Work out the finished part from the listing and answer in its coordinate system (mm). A direction names the side the tool comes from. Give positions to 0.01 mm unless a question says otherwise; leave off trailing zeros. Loops run counter-clockwise (first coordinate to the right, second up) from the corner with the lowest first, then second, coordinate; pieces in that order, holes last. Notation, with made-up numbers: (-22, 57.25) - (-2, 57.25) arc R14 ccw to (-2, 67.25) - close; hole circle Ø10 at (61.25, 20.25). An arc over 180 degrees is marked (long way). One line per item, written item: value.
from build123d import *

# Parameters (mm, degrees)
CYLINDER_R      = 1.65
CYLINDER_DEPTH  = 30
PAD005_DEPTH    = 1.05
PAD001_DEPTH    = 3.3
POCKET004_DEPTH = 28.001
PAD002_DEPTH    = 0.5
FILLET_R        = 0.7
FILLET002_R     = 1


with BuildPart() as black_led_base:
    # Cylinder → Cylinder (join)
    with BuildSketch(Plane(origin=(-6, 0, -15), x_dir=(1, 0, 0), z_dir=(0, 0, 1))):
        Circle(CYLINDER_R)
    extrude(amount=CYLINDER_DEPTH)


with BuildPart() as obj1:
    # Sketch016 → Pad005 (new body, symmetric)
    with BuildSketch(Plane.XZ):
        Polygon((-6, 2.5), (-6, -0.5), (0, -0.5), (0, 0.5), align=None)
    extrude(amount=PAD005_DEPTH, both=True)


with BuildPart() as black_d:
    # Sketch005 → Pad001 (new body, symmetric)
    with BuildSketch(Plane.XZ):
        Polygon((0, 0), (0, -2), (-5, -2), (-10, 3), (-16, 3), (-28, 5), (-28, 10), (-4, 10), (0, 4), align=None)
    extrude(amount=PAD001_DEPTH, both=True)

    # Sketch006 → Pocket004 (cut, through all)
    with BuildSketch(Plane.YZ):
        Polygon((-3.3, 0), (-3.3, 3), (0, 21.71523), (3.3, 3), (3.3, 0), (13, 0), (13, 26), (-13, 26), (-13, 0), align=None)
    extrude(amount=-POCKET004_DEPTH, mode=Mode.SUBTRACT)

    # Sketch008 → Pad002 (join, symmetric)
    with BuildSketch(Plane.XZ.offset(2)):
        with BuildLine():
            ThreePointArc((-15.5, 1.5), (-15, 1), (-14.5, 1.5))
            Line((-14.5, 1.5), (-14.5, 3))
            ThreePointArc((-14.5, 3), (-15, 3.5), (-15.5, 3))
            Line((-15.5, 1.5), (-15.5, 3))
        make_face()
        with BuildLine():
            ThreePointArc((-16.5, 3), (-17, 3.5), (-17.5, 3))
            Line((-17.5, 3), (-17.5, 1.5))
            ThreePointArc((-17.5, 1.5), (-17, 1), (-16.5, 1.5))
            Line((-16.5, 3), (-16.5, 1.5))
        make_face()
    pad002 = extrude(amount=PAD002_DEPTH, both=True)

    # Mirrored001: Pad002 across XZ
    add(pad002.mirror(Plane.XZ))

    # Fillet
    fillet_edges = [black_d.edges().sort_by_distance(p)[0] for p in [
        (0, -3.211837, 3.5),
        (0, 3.211837, 3.5),
    ]]
    fillet(fillet_edges, radius=FILLET_R)

    # Fillet002
    fillet002_edges = [black_d.edges().sort_by_distance(p)[0] for p in [
        (-28, -2.506529, 7.5),
        (-28, 2.506529, 7.5),
    ]]
    fillet(fillet002_edges, radius=FILLET002_R)

    # Boolean001: cut black_led_BASE, obj1
    add(black_led_base.part, mode=Mode.SUBTRACT)
    add(obj1.part, mode=Mode.SUBTRACT)


with BuildPart() as black_d_1:
    # Clone009 placement: moved
    add(black_d.part.moved(Location((0, 22.95, 0))))


solid = black_d_1.part
1. Section C-C (x = -17) is taken. Write down the section's boundary in (y, z).
Output:
outline: (19.68, 3.17) - (20.45, 3.17) - (20.45, 1) - (21.45, 1) - (21.45, 3.17) - (24.45, 3.17) - (24.45, 1) - (25.45, 1) - (25.45, 3.17) - (26.22, 3.17) - (25.02, 10) - (20.88, 10) - close
2. For faces 1 (the flat face through (-28, 23, 7)), 2 (the flat face through (-17, 20.45, 2)), 3 (the flat face through (-15.5, 21, 2)), 4 (the flat face through (-17, 25.45, 2)), 5 (the flat face through (-17.5, 21, 2)), determine the directions among +Z, -Z, +X, -X, +Y, -Y from which every point of the face is accessible in a straight line to the end or side of a thin tool.
Output:
face 1: +Z, -Z, -X, +Y, -Y
face 2: -Z, -X, -Y
face 3: -Z, +Y, -Y
face 4: -Z, -X, +Y
face 5: -Z, -X, +Y, -Y
3. Section A-A (y = 22.95) is taken. Write down the section's boundary in (x, z).
Output:
outline: (-28, 5) - (-16, 3) - (-10, 3) - (-7.65, 0.65) - (-7.65, 10) - (-28, 10) - close; (-4.35, -2) - (0, -2) - (0, -0.5) - (-4.35, -0.5) - close; (-4.35, 1.95) - (0, 0.5) - (0, 4) - (-4, 10) - (-4.35, 10) - close
4. Section B-B (x = -5.75) is taken. Write down the section's boundary in (y, z).
Output:
outline: (19.65, -1.25) - (21.32, -1.25) - (21.32, 10) - (20.88, 10) - (19.65, 3) - close; (24.58, -1.25) - (26.25, -1.25) - (26.25, 3) - (25.02, 10) - (24.58, 10) - close
5. Flat-ended cylindrical pins translate along their axes: pin 1 Ø2 at (x, z) = (-18, 6.5) entering from +Y; pin 2 Ø2 at (y, z) = (22.5, 8.5) entering from +X; pin 3 Ø3 at (x, y) = (-12, 22) entering from -Z. Find the tip coordinate at first contact, or state that the pin passes through.
Output:
pin 1: stops at y = 25.81
pin 2: stops at x = -2.33
pin 3: stops at z = 3
6. The mould has two halves that part along X. Classify faces 6 (the flat face through (-2, 23, 7)), 7 (the cylindrical face through (-17, 21, 1)), 8 (the flat face through (-14.5, 21, 2)), 9 (the cylindrical face through (-27.7, 20.73, 7.49)): released by +X, released by -X, zero draft, split by the parting line, or undercut.
Output:
face 6: released by +X
face 7: undercut
face 8: undercut
face 9: released by -X
7. Find the intervals of material crossed by line 1 along Y through (x, z) = (-6, 0.5); line 2 along X through (y, z) = (25, 1.5); line 3 along X through (y, z) = (22.75, 7.75), in increasing order.
Output:
line 1: y = 19.65 to 21.3, 24.6 to 26.25
line 2: x = -17.5 to -16.5, -15.5 to -14.5, -8.5 to 0
line 3: x = -28 to -7.64, -4.36 to -2.5
